The listing builds one solid part. Answer for the finished solid, in the listing's coordinates (mm). A direction names the side the tool comes from. Round coordinates to 2 decimals unless told otherwise and drop trailing zeros. Write each loop counter-clockwise with the first axis right and the second up, starting at its lowest first coordinate (ties: lowest second). Pieces come first, ordered by that corner, then holes.
from build123d import *

# Parameters (mm, degrees)
SKETCH006_R  = 0.5
PAD003_DEPTH = 0.25
BOX_W        = 11.5
BOX_H        = 5.5
BOX_DEPTH    = 1.125


with BuildPart() as pin_pad:
    # Sketch006 → Pad003 (new body, symmetric)
    with BuildSketch(Plane.XZ):
        with BuildLine():
            Line((1, -1.25), (1, -3.25))
            ThreePointArc((-1, -3.25), (0, -4.25), (1, -3.25))
            Line((-1, -3.25), (-1, -1.25))
            Line((-1, -1.25), (1, -1.25))
        make_face()
        with Locations((0, -3.25)):
            Circle(SKETCH006_R, mode=Mode.SUBTRACT)
    extrude(amount=PAD003_DEPTH, both=True)


with BuildPart() as pin_right:
    # Clone base: copy of pin-pad
    add(pin_pad.part)


with BuildPart() as pin_right_1:
    # Clone placement: moved
    add(pin_right.part.moved(Location((3, 0, 0))))


with BuildPart() as pin_left:
    # Clone001 base: copy of pin-pad
    add(pin_pad.part)


with BuildPart() as pin_left_1:
    # Clone001 placement: moved
    add(pin_left.part.moved(Location((-3, 0, 0))))


with BuildPart() as board_cube:
    # Box → Box (new body)
    with BuildSketch(Plane(origin=(-5.75, -2.75, -1.25), x_dir=(1, 0, 0), z_dir=(0, 0, 1))):
        with Locations((5.75, 2.75)):
            Rectangle(BOX_W, BOX_H)
    extrude(amount=BOX_DEPTH)


with BuildPart() as slide_switch_board:
    # Fusion base: copy of pin-pad
    add(pin_pad.part)

    # Fusion: union pin-right, pin-left, board-cube
    add(pin_right_1.part)
    add(pin_left_1.part)
    add(board_cube.part)


solid = slide_switch_board.part
1. A tool of negligible diameter and unlimited length cuts with its end or side. For faces 1 (the face through (-0.02, 0, -4.25)), 2 (the face through (-3, 0.25, -2)), 3 (the face through (3, -0.25, -2)), from which of +Z, -Z, +X, -X, +Y, -Y can it reach the whole face along a straight path? Write none if from no direction.
Geometry says:
face 1: -Z, +Y, -Y
face 2: -Z, +X, -X, +Y
face 3: -Z, +X, -X, -Y
2. For a pull along X with two mould halves and no side action, classify faces 4 (the face through (5.75, 0, -1)), 5 (the face through (-5.75, 0, -1)), 6 (the face through (3, 0.25, -2)), 7 (the face through (-0.065, 0.004, -2.754)) as released by +X, released by -X, zero draft, split by the parting line, or undercut.
Geometry says:
face 4: released by +X
face 5: released by -X
face 6: zero draft
face 7: undercut
3. Straight lines are drawn through the part: line 1 along X through (y, z) = (0, -3.3); line 2 along Z through (x, y) = (-3, 0) (3 decimals); line 3 along Z through (x, y) = (3.5, -1) (3 decimals). For each, find the intervals that lie inside material, in ascending order.
Geometry says:
line 1: x = -4 to -3.5, -2.5 to -2, -1 to -0.5, 0.5 to 1, 2 to 2.5, 3.5 to 4
line 2: z = -4.25 to -3.75, -2.75 to -0.125
line 3: z = -1.25 to -0.125
4. Given pin 1 (1.6 mm diameter, centred on x = 3.5, z = -3, fed in from +Y); pin 2 (0.6 mm diameter, centred on x = 3, z = -2.5, fed in from -Y), each flat-ended and moving along its own axis, determine where each tip first touches the part or whether it passes through.
Geometry says:
pin 1: stops at y = 0.25
pin 2: stops at y = -0.25
5. Section A-A on z = -1.55 is taken. Determine the outline of the cut face in (x, y), plus the area to 3 significant figures.
Geometry says:
outline: (-4, -0.25) - (-2, -0.25) - (-2, 0.25) - (-4, 0.25) - close; (-1, -0.25) - (1, -0.25) - (1, 0.25) - (-1, 0.25) - close; (2, -0.25) - (4, -0.25) - (4, 0.25) - (2, 0.25) - close
area: 3.00 mm2
6. Section D-D on y = 1 is taken. Determine the outline of the cut face in (x, z) (3 decimals), plus the area to 3 significant figures.
Geometry says:
outline: (-5.75, -1.25) - (5.75, -1.25) - (5.75, -0.125) - (-5.75, -0.125) - close
area: 12.9 mm2
7. Section B-B on x = -3 is taken. Determine the outline of the cut face in (y, z) (3 decimals), plus the area to 3 significant figures.
Geometry says:
outline: (-2.75, -1.25) - (-0.25, -1.25) - (-0.25, -2.75) - (0.25, -2.75) - (0.25, -1.25) - (2.75, -1.25) - (2.75, -0.125) - (-2.75, -0.125) - close; (-0.25, -4.25) - (0.25, -4.25) - (0.25, -3.75) - (-0.25, -3.75) - close
area: 7.19 mm2
8. Section C-C on z = -3 is taken. Determine the outline of the cut face in (x, y), plus the area to 3 significant figures.
Geometry says:
outline: (-4, -0.25) - (-3.43, -0.25) - (-3.43, 0.25) - (-4, 0.25) - close; (-2.57, -0.25) - (-2, -0.25) - (-2, 0.25) - (-2.57, 0.25) - close; (-1, -0.25) - (-0.43, -0.25) - (-0.43, 0.25) - (-1, 0.25) - close; (0.43, -0.25) - (1, -0.25) - (1, 0.25) - (0.43, 0.25) - close; (2, -0.25) - (2.57, -0.25) - (2.57, 0.25) - (2, 0.25) - close; (3.43, -0.25) - (4, -0.25) - (4, 0.25) - (3.43, 0.25) - close
area: 1.70 mm2
